Verification items for the finished model (mm, model axes). Face numbers are marked on the shaded views. A direction names the side the tool comes from. Coordinates: 2 decimals unless noted, no trailing zeros. Loops run counter-clockwise (first coordinate to the right, second up) from the corner with the lowest first, then second, coordinate; pieces in that order, holes last. Notation, with made-up numbers: M 27.5,19 L 56.5,19 A17 ccw 56.5,48 Z; hole C 37,-34.75 d7. An arc over 180 degrees is marked long. Write item = value, one per line. Start each with the question number.
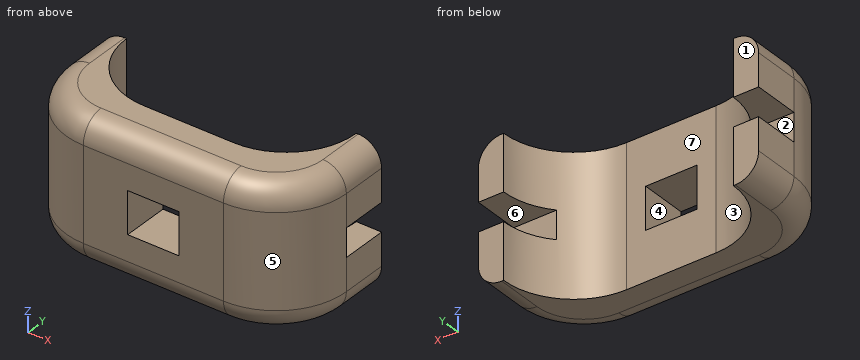
```python
from build123d import *

# Parameters (mm, degrees)
SKETCH_1_W          = 12
SKETCH_1_H          = 6
EXTRUDE_1_DEPTH     = 5
SKETCH_2_W          = 2.2
SKETCH_2_H          = 1.8
CUT_EXTRUDE_1_DEPTH = 5
FILLET_1_R          = 3
SKETCH_3_W          = 9.838074984
SKETCH_3_H          = 6
CUT_EXTRUDE_2_DEPTH = 3
FILLET_2_R          = 3
FILLET_3_R          = 1
FILLET_4_R          = 1
SKETCH_4_W          = 12
SKETCH_4_H          = 1.214577158
CUT_EXTRUDE_3_DEPTH = 2


with BuildPart() as part:
    # Эскиз1 → Бобышка-Вытянуть1 (new body)
    with BuildSketch(Plane(origin=(0, 0, 0), x_dir=(1, 0, 0), z_dir=(0, 1, 0))):
        Rectangle(SKETCH_1_W, SKETCH_1_H)
    extrude(amount=EXTRUDE_1_DEPTH)

    # Эскиз2 → Вырез-Вытянуть1 (cut)
    with BuildSketch(Plane.XZ):
        Rectangle(SKETCH_2_W, SKETCH_2_H)
    extrude(amount=-CUT_EXTRUDE_1_DEPTH, mode=Mode.SUBTRACT)

    # Скругление1
    fillet_1_edges = [part.edges().sort_by_distance(p)[0] for p in [
        (6, 0, 0),
        (-6, 0, 0),
    ]]
    fillet(fillet_1_edges, radius=FILLET_1_R)

    # Эскиз3 → Вырез-Вытянуть2 (cut)
    with BuildSketch(Plane(origin=(0, 5, 0), x_dir=(1, 0, 0), z_dir=(0, 1, 0))):
        Rectangle(SKETCH_3_W, SKETCH_3_H)
    extrude(amount=-CUT_EXTRUDE_2_DEPTH, mode=Mode.SUBTRACT)

    # Скругление2
    fillet_2_edges = [part.edges().sort_by_distance(p)[0] for p in [
        (4.919037492, 2, 0),
        (-4.919037492, 2, 0),
    ]]
    fillet(fillet_2_edges, radius=FILLET_2_R - 0.0001)  # a hair under: the kernel refuses the full size

    # Скругление3
    fillet_3_edges = [part.edges().sort_by_distance(p)[0] for p in [
        (0, 0, -3),
        (-5.121320344, 0.878679656, -3),
        (5.121320344, 0.878679656, -3),
        (-6, 4, -3),
        (6, 4, -3),
    ]]
    fillet(fillet_3_edges, radius=FILLET_3_R)

    # Скругление4
    fillet_4_edges = [part.edges().sort_by_distance(p)[0] for p in [
        (0, 0, 3),
        (-5.121320344, 0.878679656, 3),
        (5.121320344, 0.878679656, 3),
        (6, 4, 3),
        (-6, 4, 3),
    ]]
    fillet(fillet_4_edges, radius=FILLET_4_R)

    # Эскиз4 → Вырез-Вытянуть3 (cut)
    with BuildSketch(Plane(origin=(0, 5, 0), x_dir=(1, 0, 0), z_dir=(0, 1, 0))):
        Rectangle(SKETCH_4_W, SKETCH_4_H)
    extrude(amount=-CUT_EXTRUDE_3_DEPTH, mode=Mode.SUBTRACT)


solid = part.part
```
Q1. Set-up check for the marked faces 1, 2 and 3: record each of +Z, -Z, +X, -X, +Y, -Y from which the full face is reachable in a straight line by a thin tool's end or side.
Q2. Sectioned sample at B-B on y = 3.9. Record the cut outline in (x, z).
Q3. Sectioned sample at A-A on z = 0.2. Record the cut outline in (x, y).
Q4. Scan lines: L1, parallel to Z at x = -4.75, y = 3.45; L2, parallel to Y at x = -1.75, z = -0.7; L3, parallel to X at y = 3.4, z = -1.05. Record each from-to range of solid material in increasing order. Write a range as [from, to].
Q5. Mould release check, pull along X, two halves, no side actions. Record for the marked faces 4, 5, 6 and 7: +X half, -X half, draft (parallel to the pull), parting line (faces both ways), or undercut.
Q6. Gauge pin test, flat ends, axial feed: pin 1 (1 mm diameter, centred on x = -4.5, z = 1.5, fed in from -Y); pin 2 (1 mm diameter, centred on x = -4, y = 0.5, fed in from +Z); pin 3 (1 mm diameter, centred on x = -5.5, z = 0, fed in from +Y). Record the tip position at first contact, or that the pin passes through.
Q7. Sectioned sample at C-C on y = 3.15. Record the cut outline in (x, z).
Solutions:
q1.face_1 = +Z, -Z, +X, -X, +Y
q1.face_2 = +X, -X, +Y
q1.face_3 = +Z, -Z, +Y
q2.outline = M -6,-2 A1 ccw -5,-3 L -4.71,-3 L -4.71,-0.61 L -6,-0.61 Z; M -6,0.61 L -4.71,0.61 L -4.71,3 L -5,3 A1 ccw -6,2 Z; M 4.71,-3 L 5,-3 A1 ccw 6,-2 L 6,-0.61 L 4.71,-0.61 Z; M 4.71,0.61 L 6,0.61 L 6,2 A1 ccw 5,3 L 4.71,3 Z
q3.outline = M -6,3 A3 ccw -3,0 L -1.1,0 L -1.1,2 L -1.92,2 A3 cw -4.16,3 Z; M 1.1,0 L 3,0 A3 ccw 6,3 L 4.16,3 A3 cw 1.92,2 L 1.1,2 Z
q4.L1 = [-3, -0.61], [0.61, 3]
q4.L2 = [0, 2]
q4.L3 = [-6, -4.46], [4.46, 6]
q5.face_4 = undercut
q5.face_5 = +X half
q5.face_6 = draft
q5.face_7 = undercut
q6.pin_1 = 0.17
q6.pin_2 = 2.98
q6.pin_3 = 3
q7.outline = M -6,-2 A1 ccw -5,-3 L -4.28,-3 L -4.28,-0.61 L -6,-0.61 Z; M -6,0.61 L -4.28,0.61 L -4.28,3 L -5,3 A1 ccw -6,2 Z; M 4.28,-3 L 5,-3 A1 ccw 6,-2 L 6,-0.61 L 4.28,-0.61 Z; M 4.28,0.61 L 6,0.61 L 6,2 A1 ccw 5,3 L 4.28,3 Z
